Here's the drawing with two shaded views (mm, measured from the low corner). I have some questions. A direction names the side the tool comes from. Round coordinates to 2 decimals unless told otherwise and drop trailing zeros. Write each loop counter-clockwise with the first axis right and the second up, starting at its lowest first coordinate (ties: lowest second). Pieces come first, ordered by that corner, then holes. Notation, with made-up numbers: M -11,41 L 10,41 A12 ccw 10,58 Z; hole C -20,1 d1. An arc over 180 degrees is marked long. Answer as a JSON object with one key per item and string values. Group by question number.
1) Suppose I cut it at B-B, the plane y = 7.5. Write out the boundary of the cut face in (x, z), and give its area (3 significant figures).
2) I'm going to push flat-ended pins straight in: pin 1 Ø5 at (x, z) = (3.5, 14.5) entering from +Y; pin 2 Ø1.5 at (y, z) = (5, 2.5) entering from -X; pin 3 Ø1.5 at (y, z) = (1.5, 7) entering from +X. Where does each tip first touch, or does it pass through?
3) If we mould it in two halves opening along X, with no side actions, what happens to the marked faces 6, 7 and 8? For each: +X half, -X half, draft (parallel to the pull), parting line (faces both ways), or undercut.
4) Suppose I cut it at A-A, the plane z = 4.5. Write out the boundary of the cut face in (x, y).
5) On a 3-axis mill with a long thin cutter (end or side, diameter ignored), from which of +Z, -Z, +X, -X, +Y, -Y can I reach the whole of each face in a straight line? I mean the marked faces 1, 2, 3, 4 and 5. Say none if no direction works.
6) Suppose I cut it at D-D, the plane z = 2.5. State how many separate pieces and enclosed holes the cut face has, and give its area (3 significant figures).
7) Please list where these lines run through material, in increasing order: L1, parallel to X at y = 2.75, z = 9; L2, parallel to X at y = 6, z = 2.25; L3, parallel to Y at x = 21, z = 1.5. Write a range as [from, to].
8) Suppose I cut it at C-C, the plane y = 9.25. Write out the boundary of the cut face in (x, z), and give its area (3 significant figures).
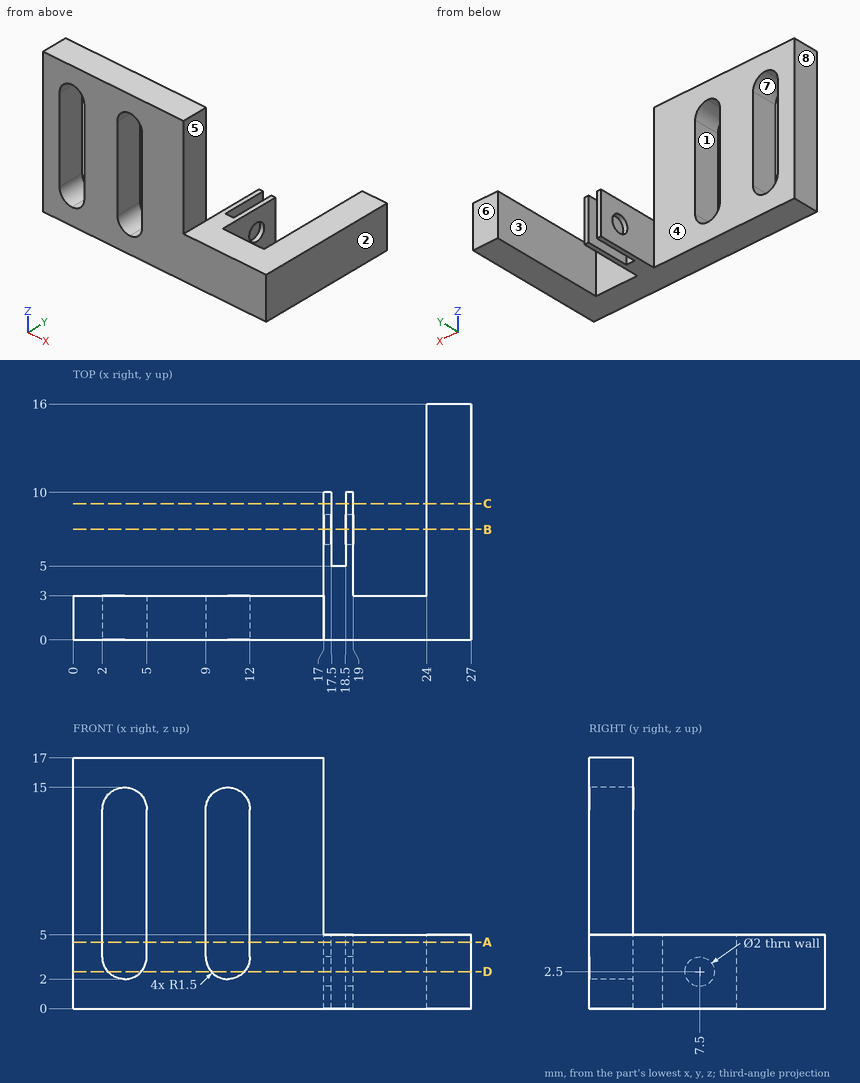
Results:
{
 "1": {"outline": "M 17,0 L 17.5,0 L 17.5,1.5 L 17,1.5 Z; M 17,3.5 L 17.5,3.5 L 17.5,5 L 17,5 Z; M 18.5,0 L 19,0 L 19,1.5 L 18.5,1.5 Z; M 18.5,3.5 L 19,3.5 L 19,5 L 18.5,5 Z; M 24,0 L 27,0 L 27,5 L 24,5 Z", "area": "18.0 mm^2"},
 "2": {"pin 1": "y = 3", "pin 2": "x = 17", "pin 3": "x = 17"},
 "3": {"face 6": "draft", "face 7": "undercut", "face 8": "-X half"},
 "4": {"outline": "M 0,0 L 2,0 L 2,3 L 0,3 Z; M 5,0 L 9,0 L 9,3 L 5,3 Z; M 12,0 L 27,0 L 27,16 L 24,16 L 24,3 L 19,3 L 19,10 L 18.5,10 L 18.5,5 L 17.5,5 L 17.5,10 L 17,10 L 17,3 L 12,3 Z"},
 "5": {"face 1": "+Y, -Y", "face 2": "+Z, -Z, +X, +Y, -Y", "face 3": "+Z, -Z, +Y", "face 4": "+Z, -Z, -X, +Y", "face 5": "+Z, +X, +Y, -Y"},
 "6": {"separate pieces": "5", "enclosed holes": "0", "area": "114 mm^2"},
 "7": {"L1": "[0, 2], [5, 9], [12, 17]", "L2": "[17, 17.5], [18.5, 19], [24, 27]", "L3": "[0, 3]"},
 "8": {"outline": "M 17,0 L 17.5,0 L 17.5,5 L 17,5 Z; M 18.5,0 L 19,0 L 19,5 L 18.5,5 Z; M 24,0 L 27,0 L 27,5 L 24,5 Z", "area": "20.0 mm^2"}
}
